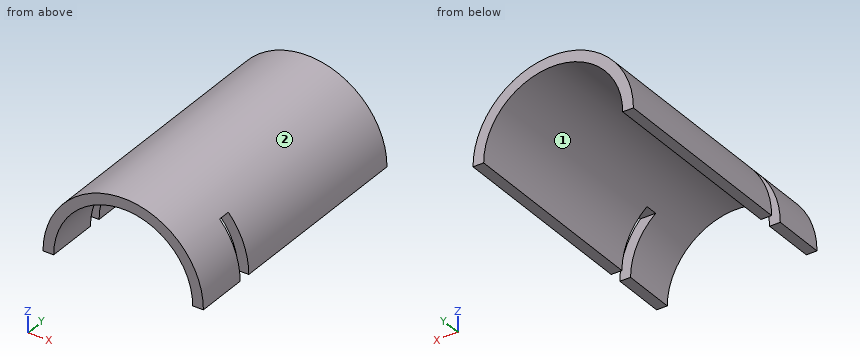
```python
from build123d import *

# Parameters (mm, degrees)
F1_DEPTH = 127
F2_W     = 6
F2_H     = 25.4
F3_DEPTH = 101.6
F4_DEPTH = 101.6


with BuildPart() as f1:
    # F0 (on Front) → F1 (new body)
    with BuildSketch(Plane.XZ):
        with BuildLine():
            Line((33.02, 0), (38.1, 0))
            ThreePointArc((38.1, 0), (0, 38.1), (-38.1, 0))
            Line((-38.1, 0), (-33.02, 0))
            ThreePointArc((-33.02, 0), (0, 33.02), (33.02, 0))
        make_face()
    extrude(amount=F1_DEPTH)

    # F2 (on Right) → F3 (cut)
    with BuildSketch(Plane.YZ):
        with Locations((-98.6, 12.7)):
            Rectangle(F2_W, F2_H)
    extrude(amount=-F3_DEPTH, mode=Mode.SUBTRACT)

    # F2 (on Right) → F4 (cut)
    with BuildSketch(Plane.YZ):
        with Locations((-98.6, 12.7)):
            Rectangle(F2_W, F2_H)
    extrude(amount=F4_DEPTH, mode=Mode.SUBTRACT)


solid = f1.part
```
Model file for the job. Use its own axes, mm. Face numbers are marked on the shaded views. Coordinates: 2 decimals unless noted, no trailing zeros. Order: outer loops, then holes, each group sorted by start corner. A loop starts at its lowest first (then second) coordinate and runs counter-clockwise, first axis right, second up. Notation, with made-up numbers: (-1.5, 34) -> (37.5, 34) arc R30 ccw to (37.5, 56) -> close; hole circle Ø7 at (-16.5, 77.5). An arc over 180 degrees is marked (long way). Answer as a JSON object with one key per item and string values. Group by question number.
1) Cut at C-C, the plane y = -47. Write the cut outline in (x, z).
2) Pull direction X, two halves, no side cores. Call the marked faces 1 and 2: +X half, -X half, draft (parallel to the pull), parting line (faces both ways), or undercut.
3) Cut at D-D, the plane x = 10. Write the cut outline in (y, z), then the cut area to 3 significant figures.
4) Drill centre lines: L1, parallel to Y at x = -27.5, z = 19; L2, parallel to X at y = -61.5, z = 15; L3, parallel to X at y = -39, z = 8. Where is each one in solid material? Low to high.
5) Cut at A-A, the plane x = 31. Write the cut outline in (y, z), then the cut area to 3 significant figures.
6) Flat gauge pins, fed straight in: pin 1 (18.5 mm diameter, centred on x = 32, z = 17.5, fed in from +Y); pin 2 (1 mm diameter, centred on y = -63, z = 9, fed in from -X); pin 3 (1.8 mm diameter, centred on x = -23, y = -98, fed in from -Z); pin 4 (10 mm diameter, centred on y = -72, z = 15, fed in from -X). Where does each tip first touch, or does it go through?
7) Cut at B-B, the plane z = 28.5. Write the cut outline in (x, y).
Check values:
{
 "1": {"outline": "(-38.1, 0) -> (-33.02, 0) arc R33.02 cw to (33.02, 0) -> (38.1, 0) arc R38.1 ccw to start"},
 "2": {"face 1": "undercut", "face 2": "parting line"},
 "3": {"outline": "(-127, 31.47) -> (0, 31.47) -> (0, 36.76) -> (-127, 36.76) -> close", "area": "672 mm²"},
 "4": {"L1": "y = -127 to -101.6, -95.6 to 0", "L2": "x = -35.02 to -29.42, 29.42 to 35.02", "L3": "x = -37.25 to -32.04, 32.04 to 37.25"},
 "5": {"outline": "(-127, 11.37) -> (-101.6, 11.37) -> (-101.6, 22.15) -> (-127, 22.15) -> close; (-95.6, 11.37) -> (0, 11.37) -> (0, 22.15) -> (-95.6, 22.15) -> close", "area": "1,300 mm²"},
 "6": {"pin 1": "stops at y = 0", "pin 2": "stops at x = -37.14", "pin 3": "stops at z = 25.4", "pin 4": "stops at x = -36.76"},
 "7": {"outline": "(-25.29, -127) -> (-16.68, -127) -> (-16.68, 0) -> (-25.29, 0) -> close; (16.68, -127) -> (25.29, -127) -> (25.29, 0) -> (16.68, 0) -> close"}
}
